```python
from build123d import *

# Parameters (mm, degrees)
SKETCH_1_W      = 960
SKETCH_1_H      = 1010
SKETCH_1_R      = 15.5
EXTRUDE_3_DEPTH = 16


with BuildPart() as part:
    # 草图1 → 拉伸3 (new body)
    with BuildSketch(Plane.XY):
        with Locations((441.964087771, -474.512070354)):
            Rectangle(SKETCH_1_W, SKETCH_1_H)
        with Locations((190.531101581, -747.31686037)):
            Circle(SKETCH_1_R, mode=Mode.SUBTRACT)
        with Locations((27.879035044, -923.794352563)):
            Circle(SKETCH_1_R, mode=Mode.SUBTRACT)
        with Locations((109.205068312, -835.555606466)):
            Circle(SKETCH_1_R, mode=Mode.SUBTRACT)
        with Locations((205.017301257, -842.265004211)):
            Circle(SKETCH_1_R, mode=Mode.SUBTRACT)
        with Locations(Location((94.718868636, -740.607462625, 0), (0, 0, 180))):
            Circle(SKETCH_1_R, mode=Mode.SUBTRACT)
        with Locations((346.964087771, -904.512070354)):
            Circle(SKETCH_1_R, mode=Mode.SUBTRACT)
        with Locations((346.964087771, -704.512070354)):
            Circle(SKETCH_1_R, mode=Mode.SUBTRACT)
        with Locations((346.964087771, -804.512070354)):
            Circle(SKETCH_1_R, mode=Mode.SUBTRACT)
        with Locations((381.964087771, -569.512070354)):
            Circle(SKETCH_1_R, mode=Mode.SUBTRACT)
        with Locations((181.964087771, -569.512070354)):
            Circle(SKETCH_1_R, mode=Mode.SUBTRACT)
        with Locations((281.964087771, -569.512070354)):
            Circle(SKETCH_1_R, mode=Mode.SUBTRACT)
        with Locations((61.964087771, -569.512070354)):
            Circle(SKETCH_1_R, mode=Mode.SUBTRACT)
        with Locations((13.392835367, -828.846208722)):
            Circle(SKETCH_1_R, mode=Mode.SUBTRACT)
        with Locations(Location((123.691267988, -930.503750308, 0), (0, 0, 180))):
            Circle(SKETCH_1_R, mode=Mode.SUBTRACT)
        with Locations((760.236907554, -930.503750308)):
            Circle(SKETCH_1_R, mode=Mode.SUBTRACT)
        with Locations(Location((870.535340175, -828.846208722, 0), (0, 0, 180))):
            Circle(SKETCH_1_R, mode=Mode.SUBTRACT)
        with Locations(Location((821.964087771, -569.512070354, 0), (0, 0, 180))):
            Circle(SKETCH_1_R, mode=Mode.SUBTRACT)
        with Locations(Location((601.964087771, -569.512070354, 0), (0, 0, 180))):
            Circle(SKETCH_1_R, mode=Mode.SUBTRACT)
        with Locations(Location((701.964087771, -569.512070354, 0), (0, 0, 180))):
            Circle(SKETCH_1_R, mode=Mode.SUBTRACT)
        with Locations(Location((501.964087771, -569.512070354, 0), (0, 0, 180))):
            Circle(SKETCH_1_R, mode=Mode.SUBTRACT)
        with Locations(Location((536.964087771, -804.512070354, 0), (0, 0, 180))):
            Circle(SKETCH_1_R, mode=Mode.SUBTRACT)
        with Locations(Location((536.964087771, -704.512070354, 0), (0, 0, 180))):
            Circle(SKETCH_1_R, mode=Mode.SUBTRACT)
        with Locations(Location((536.964087771, -904.512070354, 0), (0, 0, 180))):
            Circle(SKETCH_1_R, mode=Mode.SUBTRACT)
        with Locations((789.209306906, -740.607462625)):
            Circle(SKETCH_1_R, mode=Mode.SUBTRACT)
        with Locations(Location((678.910874285, -842.265004211, 0), (0, 0, 180))):
            Circle(SKETCH_1_R, mode=Mode.SUBTRACT)
        with Locations(Location((774.72310723, -835.555606466, 0), (0, 0, 180))):
            Circle(SKETCH_1_R, mode=Mode.SUBTRACT)
        with Locations(Location((856.049140499, -923.794352563, 0), (0, 0, 180))):
            Circle(SKETCH_1_R, mode=Mode.SUBTRACT)
        with Locations(Location((693.397073961, -747.31686037, 0), (0, 0, 180))):
            Circle(SKETCH_1_R, mode=Mode.SUBTRACT)
        with Locations((693.397073961, -201.707280338)):
            Circle(SKETCH_1_R, mode=Mode.SUBTRACT)
        with Locations((856.049140499, -25.229788144)):
            Circle(SKETCH_1_R, mode=Mode.SUBTRACT)
        with Locations((774.72310723, -113.468534241)):
            Circle(SKETCH_1_R, mode=Mode.SUBTRACT)
        with Locations((678.910874285, -106.759136496)):
            Circle(SKETCH_1_R, mode=Mode.SUBTRACT)
        with Locations(Location((789.209306906, -208.416678082, 0), (0, 0, 180))):
            Circle(SKETCH_1_R, mode=Mode.SUBTRACT)
        with Locations((536.964087771, -44.512070354)):
            Circle(SKETCH_1_R, mode=Mode.SUBTRACT)
        with Locations((536.964087771, -244.512070354)):
            Circle(SKETCH_1_R, mode=Mode.SUBTRACT)
        with Locations((536.964087771, -144.512070354)):
            Circle(SKETCH_1_R, mode=Mode.SUBTRACT)
        with Locations((501.964087771, -379.512070354)):
            Circle(SKETCH_1_R, mode=Mode.SUBTRACT)
        with Locations((701.964087771, -379.512070354)):
            Circle(SKETCH_1_R, mode=Mode.SUBTRACT)
        with Locations((601.964087771, -379.512070354)):
            Circle(SKETCH_1_R, mode=Mode.SUBTRACT)
        with Locations((821.964087771, -379.512070354)):
            Circle(SKETCH_1_R, mode=Mode.SUBTRACT)
        with Locations((870.535340175, -120.177931986)):
            Circle(SKETCH_1_R, mode=Mode.SUBTRACT)
        with Locations(Location((760.236907554, -18.520390399, 0), (0, 0, 180))):
            Circle(SKETCH_1_R, mode=Mode.SUBTRACT)
        with Locations((123.691267988, -18.520390399)):
            Circle(SKETCH_1_R, mode=Mode.SUBTRACT)
        with Locations(Location((13.392835367, -120.177931986, 0), (0, 0, 180))):
            Circle(SKETCH_1_R, mode=Mode.SUBTRACT)
        with Locations(Location((61.964087771, -379.512070354, 0), (0, 0, 180))):
            Circle(SKETCH_1_R, mode=Mode.SUBTRACT)
        with Locations(Location((281.964087771, -379.512070354, 0), (0, 0, 180))):
            Circle(SKETCH_1_R, mode=Mode.SUBTRACT)
        with Locations(Location((181.964087771, -379.512070354, 0), (0, 0, 180))):
            Circle(SKETCH_1_R, mode=Mode.SUBTRACT)
        with Locations(Location((381.964087771, -379.512070354, 0), (0, 0, 180))):
            Circle(SKETCH_1_R, mode=Mode.SUBTRACT)
        with Locations(Location((346.964087771, -144.512070354, 0), (0, 0, 180))):
            Circle(SKETCH_1_R, mode=Mode.SUBTRACT)
        with Locations(Location((346.964087771, -244.512070354, 0), (0, 0, 180))):
            Circle(SKETCH_1_R, mode=Mode.SUBTRACT)
        with Locations(Location((346.964087771, -44.512070354, 0), (0, 0, 180))):
            Circle(SKETCH_1_R, mode=Mode.SUBTRACT)
        with Locations((94.718868636, -208.416678082)):
            Circle(SKETCH_1_R, mode=Mode.SUBTRACT)
        with Locations(Location((205.017301257, -106.759136496, 0), (0, 0, 180))):
            Circle(SKETCH_1_R, mode=Mode.SUBTRACT)
        with Locations(Location((109.205068312, -113.468534241, 0), (0, 0, 180))):
            Circle(SKETCH_1_R, mode=Mode.SUBTRACT)
        with Locations(Location((27.879035044, -25.229788144, 0), (0, 0, 180))):
            Circle(SKETCH_1_R, mode=Mode.SUBTRACT)
        with Locations(Location((190.531101581, -201.707280338, 0), (0, 0, 180))):
            Circle(SKETCH_1_R, mode=Mode.SUBTRACT)
    extrude(amount=EXTRUDE_3_DEPTH)


solid = part.part
```
Verification items for the finished model (mm, model axes). Round coordinates to 2 decimals unless told otherwise and drop trailing zeros. Order: outer loops, then holes, each group sorted by start corner. A loop starts at its lowest first (then second) coordinate and runs counter-clockwise, first axis right, second up. Notation, with made-up numbers: (44, 36.5) - (48, 36.5) arc R30 ccw to (48, 73.5) - close; hole circle Ø9 at (-19, -36). An arc over 180 degrees is marked (long way). Use CSV: the item, a comma, the result in double quotes.
(1) Gauge pin test, flat end, axial feed: pin 1 Ø18.5 at (x, y) = (190.53, -747.32) entering from +Z. Record the tip position at first contact, or that the pin passes through.
Entries:
pin 1,"through"
(2) Mould release check, pull along Y, two halves, no side actions. Record for faces 1 (the face through (190.297, -556.442, 7.888)), 2 (the face through (505.32, -554.38, 7.89)): released by +Y, released by -Y, zero draft, split by the parting line, or undercut.
Entries:
face 1,"undercut"
face 2,"undercut"
(3) Thickness scan on probe 1 along Y at (x, z) = (113, 7.25); probe 2 along Y at (x, z) = (71, 7.5); probe 3 along Y at (x, z) = (56, 8.5). Record the ranges inside material, lowest first. Write a range as from..to.
Entries:
probe 1,"-979.51..-941.73, -919.28..-850.58, -820.53..-128.5, -98.44..-29.74, -7.3..30.49"
probe 2,"-979.51..-582.11, -556.92..-392.11, -366.92..30.49"
probe 3,"-979.51..-583.82, -555.21..-393.82, -365.21..30.49"
(4) Section check A-A on x = 821.5. Record the boundary of the cut face in (y, z), and give its area (3 significant figures).
Entries:
outline,"(-979.51, 0) - (-585.01, 0) - (-585.01, 16) - (-979.51, 16) - close; (-554.02, 0) - (-395.01, 0) - (-395.01, 16) - (-554.02, 16) - close; (-364.02, 0) - (30.49, 0) - (30.49, 16) - (-364.02, 16) - close"
area,"15,200 mm^2"
(5) Section check B-B on z = 7. State how many separate pieces and enclosed holes the cut face has, and give its area (3 significant figures).
Entries:
separate pieces,"1"
enclosed holes,"56"
area,"927,000 mm^2"
